from build123d import *

# Parameters (mm, degrees)
EXTRUSION1_DEPTH = 325
ESQUISSE3_R      = 1.5
ESQUISSE3_R_2    = 2
EXTRUSION3_DEPTH = 300
ESQUISSE4_R      = 1.5
EXTRUSION5_DEPTH = 10


with BuildPart() as part:
    # Esquisse1 → Extrusion1 (new body)
    with BuildSketch(Plane.XY):
        Polygon((-17.43168638, 4.773368421), (-17.43168638, -15.226631579), (2.56831362, -15.226631579), (2.56831362, -13.726631579), (-15.93168638, -13.726631579), (-15.93168638, 4.773368421), align=None)
    extrude(amount=EXTRUSION1_DEPTH)

    # Esquisse3 → Extrusion3 (cut)
    with BuildSketch(Plane(origin=(-15.93168638, 0, 0), x_dir=(0, 0, -1), z_dir=(1, 0, 0))):
        with Locations((-316.5, -5.226631579)):
            Circle(ESQUISSE3_R)
        with Locations((-8.5, -5.226631579)):
            Circle(ESQUISSE3_R)
        with Locations((-35, -7.726631579)):
            Circle(ESQUISSE3_R_2)
        with Locations((-46, -7.726631579)):
            Circle(ESQUISSE3_R_2)
        with Locations((-290, -7.726631579)):
            Circle(ESQUISSE3_R_2)
        with Locations((-279, -7.726631579)):
            Circle(ESQUISSE3_R_2)
        with Locations((-235, -5.226631579)):
            Circle(ESQUISSE3_R)
        with Locations((-90, -5.226631579)):
            Circle(ESQUISSE3_R)
    extrude(amount=-EXTRUSION3_DEPTH, mode=Mode.SUBTRACT)

    # Esquisse4 → Extrusion5 (cut)
    with BuildSketch(Plane.XZ.offset(15.226631579)):
        with Locations(Location((-7.43168638, 235, 0), (0, 0, 270))):
            Circle(ESQUISSE4_R)
    extrude(amount=-EXTRUSION5_DEPTH, mode=Mode.SUBTRACT)


solid = part.part
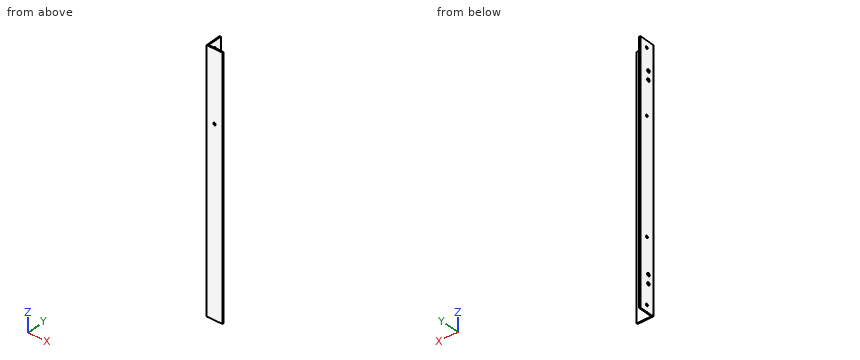
Check sheet for the modelled part. Datum: model origin and axes. Units: mm. Coordinates: 2 decimals unless noted, no trailing zeros. Loops run counter-clockwise (first coordinate to the right, second up) from the corner with the lowest first, then second, coordinate; pieces in that order, holes last. Notation, with made-up numbers: (-33.75, 65) -> (18.25, 65) arc R8 ccw to (18.25, 74) -> close; hole circle Ø2 at (42.5, 83). An arc over 180 degrees is marked (long way). Answer in a Markdown table with one row per item.
1. Sectioned sample at B-B, the plane y = -0.5. Record the boundary of the cut face in (x, z).
Check values:
| item | result |
|---|---|
| outline | (-17.43, 0) -> (-15.93, 0) -> (-15.93, 325) -> (-17.43, 325) -> close |
2. Sectioned sample at A-A, the plane z = 252. Record the boundary of the cut face in (x, y).
Check values:
| item | result |
|---|---|
| outline | (-17.43, -15.23) -> (2.57, -15.23) -> (2.57, -13.73) -> (-15.93, -13.73) -> (-15.93, 4.77) -> (-17.43, 4.77) -> close |
3. Material ranges on line 1 along Z through (x, y) = (-16.5, -5); line 2 along Y through (x, z) = (-16.25, 90); line 3 along X through (y, z) = (-6.75, 155), recorded low to high. Write a range as [from, to].
Check values:
| item | result |
|---|---|
| line 1 | z = [0, 7.02], [9.98, 88.52], [91.48, 233.52], [236.48, 315.02], [317.98, 325] |
| line 2 | y = [-15.23, -6.73], [-3.73, 4.77] |
| line 3 | x = [-17.43, -15.93] |
4. Sectioned sample at C-C, the plane x = -11.75. Record the boundary of the cut face in (y, z).
Check values:
| item | result |
|---|---|
| outline | (-15.23, 0) -> (-13.73, 0) -> (-13.73, 325) -> (-15.23, 325) -> close |
5. Go/stop test with a flat-tipped pin: pin 1 (8 mm diameter, centred on x = -15, z = 77, fed in from +Y). Record where the tip stops, or that it passes through.
Check values:
| item | result |
|---|---|
| pin 1 | stops at y = 4.77 |
